```python
from build123d import *

# Parameters (mm, degrees)
F2_R            = 6.35
F3_DEPTH        = 19.051
F3_COPIES_COUNT = 4
F4_R            = 3.048


# Not quite as in the source:
# - a pattern or mirror of a feature is missing from the dataset's text; its kind, count and spacing are read off the source's solid


with BuildPart() as f1:
    # F0 (on Front) → F1 (revolve)
    with BuildSketch(Plane.XZ):
        Polygon((0, 35.052), (0, 19.05), (53.848, 19.05), (53.848, 69.85), (34.798, 69.85), (34.798, 35.052), align=None)
    revolve(axis=Axis((26.924, 0, 0), (1, 0, 0)))

    # F2 (on face) → F3 (cut, through all)
    with BuildSketch(Plane(origin=(34.798, 0, 0), x_dir=(0, -1, 0), z_dir=(-1, 0, 0))):
        with Locations((0, 53.848)):
            Circle(F2_R)
    f3 = extrude(amount=-F3_DEPTH, mode=Mode.SUBTRACT)

    # F3_copies: F3 ×4 about axis
    f3_copies_axis = Axis((0, 0, 0), (1, 0, 0))
    for i in range(1, F3_COPIES_COUNT):
        add(f3.rotate(f3_copies_axis, i * 360 / F3_COPIES_COUNT), mode=Mode.SUBTRACT)

    # F4
    f4_edges = [f1.edges().sort_by_distance(p)[0] for p in [
        (0, 0, -35.052),
        (34.798, 0, -69.85),
    ]]
    fillet(f4_edges, radius=F4_R)


solid = f1.part
```
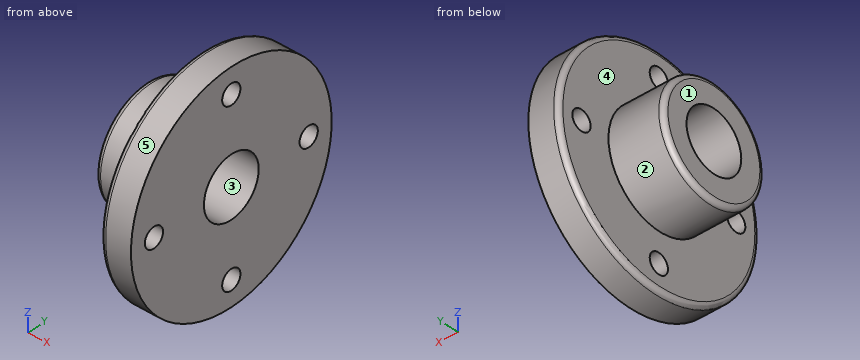
Model file for the job. Use its own axes, mm. Face numbers are marked on the shaded views. A direction names the side the tool comes from. Coordinates: 2 decimals unless noted, no trailing zeros. Order: outer loops, then holes, each group sorted by start corner. A loop starts at its lowest first (then second) coordinate and runs counter-clockwise, first axis right, second up. Notation, with made-up numbers: (50, -40) - (62, -40) arc R15 cw to (62, -34) - close; hole circle Ø9 at (-23.75, 2). An arc over 180 degrees is marked (long way). Return JSON: item names as keys, results as strings. Group by question number.
1) Saw through at A-A, the plane z = 0. Write the cut outline in (x, y).
2) Flat gauge pins, fed straight in: P1, Ø8, axis at x = 25.5, y = 27.5, coming from the +Z side; P2, Ø10, axis at x = 31.5, y = 45, coming from the -Z side; P3, Ø1.5, axis at x = 26.5, y = -6.5, coming from the -Z side. Where does each tip first touch, or does it go through?
3) Saw through at D-D, the plane x = 46. Write the cut outline in (y, z), plus the area to 3 significant figures.
4) Probe line 1 (Z direction, x = 49, y = 0); line 2 (Y direction, x = 22.5, z = 0). List the from-to ranges inside material, lowest first. Write a range as from..to.
5) Tool access for the marked faces 4 and 5: list every direction of +Z, -Z, +X, -X, +Y, -Y with a clear straight run to the whole face (end or side of a thin tool).
6) Saw through at C-C, the plane x = 17. Write the cut outline in (y, z).
7) Mould opens along Z. For the marked faces 1, 2 and 3 say: released by +Z, released by -Z, zero draft, split by the parting line, or undercut.
Values found:
{
 "1": {"outline": "(0, -32) arc R3.05 ccw to (3.05, -35.05) - (34.8, -35.05) - (34.8, -47.5) - (53.85, -47.5) - (53.85, -19.05) - (0, -19.05) - close; (0, 19.05) - (53.85, 19.05) - (53.85, 47.5) - (34.8, 47.5) - (34.8, 35.05) - (3.05, 35.05) arc R3.05 ccw to (0, 32) - close; (34.8, -66.8) arc R3.05 ccw to (37.85, -69.85) - (53.85, -69.85) - (53.85, -60.2) - (34.8, -60.2) - close; (34.8, 60.2) - (53.85, 60.2) - (53.85, 69.85) - (37.85, 69.85) arc R3.05 ccw to (34.8, 66.8) - close"},
 "2": {"P1": "stops at z = 26.01", "P2": "stops at z = -54.48", "P3": "stops at z = -34.58"},
 "3": {"outline": "circle Ø139.7 at (0, 0); hole circle Ø12.7 at (-53.85, 0); hole circle Ø38.1 at (0, 0); hole circle Ø12.7 at (0, -53.85); hole circle Ø12.7 at (0, 53.85); hole circle Ø12.7 at (53.85, 0)", "area": "13,700 mm²"},
 "4": {"line 1": "z = -69.85..-60.2, -47.5..-19.05, 19.05..47.5, 60.2..69.85", "line 2": "y = -35.05..-19.05, 19.05..35.05"},
 "5": {"face 4": "-X", "face 5": "+X, -X"},
 "6": {"outline": "circle Ø70.1 at (0, 0); hole circle Ø38.1 at (0, 0)"},
 "7": {"face 1": "zero draft", "face 2": "split by the parting line", "face 3": "undercut"}
}
